Can you work these out from the model? Positions are in its coordinate system, mm. A direction names the side the tool comes from. Give positions to 0.01 mm unless a question says otherwise; leave off trailing zeros. Loops run counter-clockwise (first coordinate to the right, second up) from the corner with the lowest first, then second, coordinate; pieces in that order, holes last. Notation, with made-up numbers: (-23.5, -37) - (-5.5, -37) arc R20 ccw to (-5.5, -3) - close; hole circle Ø2 at (47, -21). An arc over 180 degrees is marked (long way). Write item = value, one per line.
from build123d import *

# Parameters (mm, degrees)
SKETCH_1_W          = 60
SKETCH_1_H          = 42
EXTRUDE_1_DEPTH     = 1.5
SKETCH_2_W          = 18
SKETCH_2_H          = 1.5
EXTRUDE_2_DEPTH     = 1.5
SKETCH_3_W          = 12
SKETCH_3_H          = 12
CUT_EXTRUDE_1_DEPTH = 74.254692682
EXTRUDE_1_2_DEPTH   = 1.5
SKETCH_5_W          = 6.5
SKETCH_5_H          = 6.698076211
SKETCH_5_W_2        = 2.5
SKETCH_5_H_2        = 3.698076211
EXTRUDE_3_DEPTH     = 2.5
SKETCH_7_W          = 4
SKETCH_7_H          = 2.5
EXTRUDE_4_DEPTH     = 3


with BuildPart() as part:
    # Эскиз1 → Extrude 1 (new body)
    with BuildSketch(Plane(origin=(0, 0, 0), x_dir=(1, 0, 0), z_dir=(0, 1, 0))):
        with Locations((-30, 21)):
            Rectangle(SKETCH_1_W, SKETCH_1_H)
    extrude(amount=EXTRUDE_1_DEPTH)

    # Эскиз2 → Бобышка-Вытянуть2 (add, through all)
    with BuildSketch(Plane(origin=(0, 0, 0), x_dir=(1, 0, 0), z_dir=(0, 1, 0))):
        with Locations((-51, -0.75)):
            Rectangle(SKETCH_2_W, SKETCH_2_H)
    extrude(amount=EXTRUDE_2_DEPTH)

    # Эскиз3 → Вырез-Вытянуть1 (cut, through all)
    with BuildSketch(Plane(origin=(0, 0, 0), x_dir=(1, 0, 0), z_dir=(0, 1, 0))):
        with Locations((-51, 9)):
            Rectangle(SKETCH_3_W, SKETCH_3_H)
    extrude(amount=CUT_EXTRUDE_1_DEPTH, mode=Mode.SUBTRACT)

    # Эскиз4 → Extrude 1 2 (add, through all)
    with BuildSketch(Plane(origin=(0, 0, 0), x_dir=(1, 0, 0), z_dir=(0, 1, 0))):
        Polygon((-51.242640687, 1), (-43, 9.242640687), (-41.939339828, 8.181980515), (-50.181980515, -0.060660172), align=None)
        Polygon((-55.485281374, 1), (-43, 13.485281374), (-41.939339828, 12.424621202), (-54.424621202, -0.060660172), align=None)
        Polygon((-59, 1.727922061), (-43, 17.727922061), (-41.939339828, 16.66726189), (-57.939339828, 0.66726189), align=None)
        Polygon((-59, 5.970562748), (-43, 21.970562748), (-41.939339828, 20.909902577), (-57.939339828, 4.909902577), align=None)
        Polygon((-59, 10.213203436), (-52.213203436, 17), (-51.152543264, 15.939339828), (-57.939339828, 9.152543264), align=None)
    extrude(amount=EXTRUDE_1_2_DEPTH)

    # Эскиз5 → Бобышка-Вытянуть3 (add)
    with BuildSketch(Plane(origin=(0, 0, -42), x_dir=(-1, 0, 0), z_dir=(0, 0, -1))):
        with Locations((54, 4.849038106)):
            Rectangle(SKETCH_5_W, SKETCH_5_H)
        with Locations((54, 4.349038106)):
            Rectangle(SKETCH_5_W_2, SKETCH_5_H_2, mode=Mode.SUBTRACT)
    extrude(amount=-EXTRUDE_3_DEPTH)

    # Эскиз7 → Бобышка-Вытянуть4 (add)
    with BuildSketch(Plane(origin=(0, 1.5, 0), x_dir=(1, 0, 0), z_dir=(0, 1, 0))):
        with Locations((-2, 1.25)):
            Rectangle(SKETCH_7_W, SKETCH_7_H)
        with Locations((-2, 40.75)):
            Rectangle(SKETCH_7_W, SKETCH_7_H)
    extrude(amount=EXTRUDE_4_DEPTH)


solid = part.part
Q1. Imagine slicing it at B-B, the plane z = -4.5. Write out the boundary of the cut face in (x, y).
Output:
outline = (-60, 0) - (-57, 0) - (-57, 1.5) - (-60, 1.5) - close; (-56.23, 0) - (-54.11, 0) - (-54.11, 1.5) - (-56.23, 1.5) - close; (-51.99, 0) - (-49.86, 0) - (-49.86, 1.5) - (-51.99, 1.5) - close; (-47.74, 0) - (-45.62, 0) - (-45.62, 1.5) - (-47.74, 1.5) - close; (-45, 0) - (0, 0) - (0, 1.5) - (-45, 1.5) - close
Q2. For pin 1 (1.2 mm diameter, centred on x = -3, z = -1, fed in from +Y); pin 2 (2 mm diameter, centred on y = 4.5, z = -41, fed in from -X); pin 3 (3 mm diameter, centred on x = -54, y = 4, fed in from +Z), each with a flat end and sliding along its axis, tell me the tip position at first contact or that it passes through.
Output:
pin_1 = 4.5
pin_2 = -57.25
pin_3 = -39.5
Q3. Imagine slicing it at A-A, the plane y = 3.5. Write out the boundary of the cut face in (x, z), then the cut area to 3 significant figures.
Output:
outline = (-57.25, -42) - (-55.25, -42) - (-55.25, -39.5) - (-57.25, -39.5) - close; (-52.75, -42) - (-50.75, -42) - (-50.75, -39.5) - (-52.75, -39.5) - close; (-4, -42) - (0, -42) - (0, -39.5) - (-4, -39.5) - close; (-4, -2.5) - (0, -2.5) - (0, 0) - (-4, 0) - close
area = 30.0 mm2
Q4. Imagine slicing it at C-C, the plane x = -38.5. Write out the boundary of the cut face in (y, z).
Output:
outline = (0, -42) - (1.5, -42) - (1.5, 0) - (0, 0) - close
Q5. Imagine slicing it at D-D, the plane y = 7. Write out the boundary of the cut face in (x, z), then the cut area to 4 significant figures.
Output:
outline = (-57.25, -42) - (-50.75, -42) - (-50.75, -39.5) - (-57.25, -39.5) - close
area = 16.25 mm2
Q6. We'd pull the mould along Y, two halves only. Please class faces 4 (the flat face through (-54, 8.198, -41)), 5 (the flat face through (-54, 6.198, -41)), 6 (the flat face through (-17, 1, 0)): released by +Y, released by -Y, zero draft, split by the parting line, or undercut.
Output:
face_4 = released by +Y
face_5 = undercut
face_6 = zero draft
Q7. I need wall thicknesses on L1, parallel to Z at x = -52.5, y = 3; L2, parallel to Y at x = -39.5, z = -15; L3, parallel to Z at x = -14.5, y = 0.75. Which ranges of each line are inside material? Lowest first, please.
Output:
L1 = -42 to -39.5
L2 = 0 to 1.5
L3 = -42 to 0
Q8. Which directions (+Z, -Z, +X, -X, +Y, -Y) give clear straight access to the entire face, cutting with the end or side of a thin tool? Please do faces 1 (the flat face through (-53.53, 0.74, -11.44)), 2 (the flat face through (0, 1, -16)), 3 (the flat face through (-4, 3, -41)).
Output:
face_1 = +Y, -Y
face_2 = +Z, -Z, +X, +Y, -Y
face_3 = +Z, -Z, +Y
